Input: part model. Units: mm. Frame: model coordinates. Give positions to 0.01 mm unless a question says otherwise; leave off trailing zeros. Write each loop counter-clockwise with the first axis right and the second up, starting at its lowest first coordinate (ties: lowest second). Pieces come first, ordered by that corner, then holes. Notation, with made-up numbers: (-34, -35) - (1, -35) arc R24 ccw to (1, -7) - close; hole circle Ø2 at (83, 28). An arc over 180 degrees is marked (long way). Answer as CSV lines item,"result".
```python
from build123d import *

# Parameters (mm, degrees)
SKETCH1_R            = 44.45
BOSS_EXTRUDE1_DEPTH  = 2.38125
CUT_EXTRUDE1_DEPTH   = 64.041941644
SKETCH3_R            = 1.905
MOUNTING_HOLES_DEPTH = 50.924287989


with BuildPart() as part:
    # Sketch1 → Boss-Extrude1 (new, symmetric)
    with BuildSketch(Plane(origin=(0, 0, 0), x_dir=(0, 0, -1), z_dir=(1, 0, 0))):
        with Locations(Location((0, 0, 0), (0, 0, 180))):
            Circle(SKETCH1_R)
    extrude(amount=BOSS_EXTRUDE1_DEPTH, both=True)

    # Sketch2 → Cut-Extrude1 (cut, through all)
    with BuildSketch(Plane(origin=(2.38125, 0, 0), x_dir=(0, 0, -1), z_dir=(1, 0, 0))):
        with BuildLine():
            ThreePointArc((-7.937372074, -20.759305132), (0, -22.225), (7.937372074, -20.759305132))
            ThreePointArc((7.937372074, -20.759305132), (23.369671575, -18.290437479), (38.494829198, -22.225))
            ThreePointArc((38.494829198, -22.225), (0, -44.45), (-38.494829198, -22.225))
            ThreePointArc((-38.494829198, -22.225), (-23.369671575, -18.290437479), (-7.937372074, -20.759305132))
        make_face()
        with BuildLine():
            ThreePointArc((-38.494829198, 22.225), (-23.369671575, 18.290437479), (-7.937372074, 20.759305132))
            ThreePointArc((-7.937372074, 20.759305132), (0, 22.225), (7.937372074, 20.759305132))
            ThreePointArc((7.937372074, 20.759305132), (23.369671575, 18.290437479), (38.494829198, 22.225))
            ThreePointArc((38.494829198, 22.225), (0, 44.45), (-38.494829198, 22.225))
        make_face()
    extrude(amount=-CUT_EXTRUDE1_DEPTH, mode=Mode.SUBTRACT)

    # Sketch3 → Mounting holes (cut, through all)
    with BuildSketch(Plane(origin=(2.38125, 0, 0), x_dir=(0, 0, -1), z_dir=(1, 0, 0))):
        with Locations((-14.2875, 0)):
            Circle(SKETCH3_R)
        with Locations((-7.14375, 12.373337957)):
            Circle(SKETCH3_R)
        with Locations((7.14375, 12.373337957)):
            Circle(SKETCH3_R)
        with Locations((14.2875, 0)):
            Circle(SKETCH3_R)
        with Locations((7.14375, -12.373337957)):
            Circle(SKETCH3_R)
        with Locations((-7.14375, -12.373337957)):
            Circle(SKETCH3_R)
    extrude(amount=-MOUNTING_HOLES_DEPTH, mode=Mode.SUBTRACT)


solid = part.part
```
Item 1: Ray query, line 1 (Z direction, x = -1.2, y = 11); line 2 (Z direction, x = 2.2, y = -1); line 3 (Y direction, x = -0.7, z = -13). Return the intervals inside material, ascending. Write a range as from..to.
The answers:
line 1,"-43.07..-8.46, -5.82..5.82, 8.46..43.07"
line 2,"-44.44..-15.91, -12.67..12.67, 15.91..44.44"
line 3,"-19.22..-1.4, 1.4..19.22"
Item 2: Cut plane C-C on z = -28.5. Return the cut outline in (x, y), plus the area to 3 significant figures.
The answers:
outline,"(-2.38, -18.89) - (2.38, -18.89) - (2.38, 18.89) - (-2.38, 18.89) - close"
area,"180 mm²"
Item 3: Cut plane A-A on y = 0. Return the cut outline in (x, z), plus the area to 3 significant figures.
The answers:
outline,"(-2.38, -44.45) - (2.38, -44.45) - (2.38, -16.19) - (-2.38, -16.19) - close; (-2.38, -12.38) - (2.38, -12.38) - (2.38, 12.38) - (-2.38, 12.38) - close; (-2.38, 16.19) - (2.38, 16.19) - (2.38, 44.45) - (-2.38, 44.45) - close"
area,"387 mm²"
Item 4: Contact query for flat-ended pins moving along their axis: pin 1 (1 mm diameter, centred on x = 1.5, z = 14, fed in from -Y); pin 2 (2.5 mm diameter, centred on y = -12.37, z = 7.14, fed in from -X). Output: stop coordinate, or through.
The answers:
pin 1,"y = -19.11"
pin 2,"through"
Item 5: Cut plane B-B on x = -0.75. Count the separate pieces of the cut face and the enclosed holes in it, plus the area to 3 significant figures.
The answers:
separate pieces,"1"
enclosed holes,"6"
area,"3,340 mm²"
Item 6: Mould query, pull axis Z, two halves, no side actions, for faces 1 (the face through (0.03, -14.06, 6.26)), 2 (the face through (-2.381, 0, -1)), 3 (the face through (0.03, -0.33, -44.45)). Classes: +Z half, -Z half, draft (parallel to the pull), parting line (faces both ways), or undercut.
The answers:
face 1,"undercut"
face 2,"draft"
face 3,"-Z half"
Item 7: Cut plane D-D on y = -17. Return the cut outline in (x, z).
The answers:
outline,"(-2.38, -41.07) - (2.38, -41.07) - (2.38, 41.07) - (-2.38, 41.07) - close"
